CAD build for the part. Positions are in the model's coordinates, mm. Face numbers are marked on the shaded views. A direction names the side the tool comes from. Give positions to 0.01 mm unless a question says otherwise; leave off trailing zeros. Write each loop counter-clockwise with the first axis right and the second up, starting at its lowest first coordinate (ties: lowest second). Pieces come first, ordered by that corner, then holes. Notation, with made-up numbers: (13, 24) - (18, 24) arc R16 ccw to (18, 39) - close; hole circle Ø7 at (63.25, -38). An arc over 180 degrees is marked (long way). Answer as a JSON object with one key per item and string values.
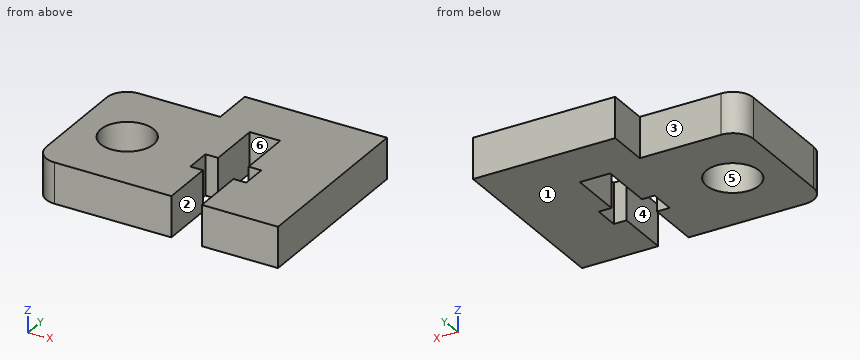
from build123d import *

# Parameters (mm, degrees)
EXTRUDE_1_DEPTH     = 4
SKETCH_2_R          = 2.6
CUT_EXTRUDE_1_DEPTH = 10


with BuildPart() as part:
    # Эскиз1 → Бобышка-Вытянуть1 (new body)
    with BuildSketch(Plane.XY):
        with BuildLine():
            Line((14, 0), (14, 18.074674191))
            Line((14, 18.074674191), (5, 18.074674191))
            Line((5, 18.074674191), (0, 18.074674191))
            Line((0, 18.074674191), (0, 14))
            Line((0, 14), (-8, 14))
            ThreePointArc((-8, 14), (-9.414213562, 13.414213562), (-10, 12))
            Line((-10, 12), (-10, 2))
            ThreePointArc((-10, 2), (-9.414213562, 0.585786438), (-8, 0))
            Line((-8, 0), (0, 0))
            Line((0, 0), (3.5, 0))
            Line((3.5, 0), (3.5, 5.25))
            Line((3.5, 5.25), (2.25, 5.25))
            Line((2.25, 5.25), (2.25, 7.75))
            Line((2.25, 7.75), (3.5, 7.75))
            Line((3.5, 7.75), (3.5, 13))
            Line((3.5, 13), (6.5, 13))
            Line((6.5, 13), (6.5, 7.75))
            Line((6.5, 7.75), (7.75, 7.75))
            Line((7.75, 7.75), (7.75, 5.25))
            Line((7.75, 5.25), (6.5, 5.25))
            Line((6.5, 5.25), (6.5, 0))
            Line((6.5, 0), (14, 0))
        make_face()
    extrude(amount=EXTRUDE_1_DEPTH)

    # Эскиз2 → Вырез-Вытянуть1 (cut)
    with BuildSketch(Plane.XY.offset(4)):
        with Locations((-5, 7)):
            Circle(SKETCH_2_R)
    extrude(amount=-CUT_EXTRUDE_1_DEPTH, mode=Mode.SUBTRACT)


solid = part.part
Item 1: Cut at A-A (y = 6). Give the cut face in (x, z), and give its area (3 significant figures).
Entries:
{"outline": "(-10, 0) - (-7.4, 0) - (-7.4, 4) - (-10, 4) - close; (-2.6, 0) - (2.25, 0) - (2.25, 4) - (-2.6, 4) - close; (7.75, 0) - (14, 0) - (14, 4) - (7.75, 4) - close", "area": "54.8 mm2"}
Item 2: Cut at C-C (z = 1). Give the cut face in (x, y).
Entries:
{"outline": "(-10, 2) arc R2 ccw to (-8, 0) - (3.5, 0) - (3.5, 5.25) - (2.25, 5.25) - (2.25, 7.75) - (3.5, 7.75) - (3.5, 13) - (6.5, 13) - (6.5, 7.75) - (7.75, 7.75) - (7.75, 5.25) - (6.5, 5.25) - (6.5, 0) - (14, 0) - (14, 18.07) - (0, 18.07) - (0, 14) - (-8, 14) arc R2 ccw to (-10, 12) - close; hole circle Ø5.2 at (-5, 7)"}
Item 3: Cut at B-B (x = 7.5). Give the cut face in (y, z).
Entries:
{"outline": "(0, 0) - (5.25, 0) - (5.25, 4) - (0, 4) - close; (7.75, 0) - (18.07, 0) - (18.07, 4) - (7.75, 4) - close"}
Item 4: Probe line 1 (Y direction, x = -5, z = 1.9); line 2 (X direction, y = 8.25, z = 2.05); line 3 (X direction, y = 5.5, z = 2.15). List the from-to ranges inside material, lowest first. Write a range as from..to.
Entries:
{"line 1": "0..4.4, 9.6..14", "line 2": "-10..-7.28, -2.72..3.5, 6.5..14", "line 3": "-10..-7.12, -2.88..2.25, 7.75..14"}
Item 5: Which spindle directions (+Z, -Z, +X, -X, +Y, -Y) get a long thin tool onto all of the face, cutting with end or side? Do the marked faces 1, 2 and 3. Say none if no direction does.
Entries:
{"face 1": "-Z, +X, -X, +Y, -Y", "face 2": "+Z, -Z, -Y", "face 3": "+Z, -Z, -X, +Y"}
Item 6: Cut at D-D (y = 3.25). Give the cut face in (x, z).
Entries:
{"outline": "(-10, 0) - (3.5, 0) - (3.5, 4) - (-10, 4) - close; (6.5, 0) - (14, 0) - (14, 4) - (6.5, 4) - close"}
Item 7: Flat gauge pin, fed straight in: P1, Ø1.2, axis at x = -6, z = 1.5, coming from the +Y side. Where does the tip first touch, or does it go through?
Entries:
{"P1": "y = 14"}
Item 8: Mould opens along Y. For the marked faces 4, 5 and 6 say: +Y half, -Y half, draft (parallel to the pull), parting line (faces both ways), or undercut.
Entries:
{"face 4": "draft", "face 5": "undercut", "face 6": "-Y half"}
